```python
from build123d import *

# Parameters (mm, degrees)
SKETCH3_R          = 8.5
SKETCH2_R          = 7.5
SKETCH4_W          = 13.98
SKETCH4_H          = 8.5
CUT_EXTRUDE1_DEPTH = 10
CUT_EXTRUDE2_DEPTH = 10
SKETCH6_R          = 1.25
CUT_EXTRUDE3_DEPTH = 10
CUT_EXTRUDE4_DEPTH = 12
FILLET1_R          = 1


with BuildPart() as part:
    # Sketch3 → Loft1 section 0
    with BuildSketch(Plane(origin=(0, 0, 0), x_dir=(0, 0, -1), z_dir=(1, 0, 0))):
        Circle(SKETCH3_R)
    # Sketch2 → Loft1 section 1
    with BuildSketch(Plane(origin=(-22, 0, 0), x_dir=(0, 0, -1), z_dir=(1, 0, 0))):
        Circle(SKETCH2_R)
    loft()

    # Sketch4 → Cut-Extrude1 (cut, symmetric)
    with BuildSketch(Plane.XY):
        with Locations((-17.99, 0)):
            Rectangle(SKETCH4_W, SKETCH4_H)
    extrude(amount=CUT_EXTRUDE1_DEPTH, both=True, mode=Mode.SUBTRACT)

    # Sketch5 → Cut-Extrude2 (cut, symmetric)
    with BuildSketch(Plane(origin=(0, 0, 0), x_dir=(1, 0, 0), z_dir=(0, 1, 0))):
        with BuildLine():
            Line((-23, -6.043769414), (-23.024844237, -1.493837243))
            ThreePointArc((-23.024844237, -1.493837243), (-21.216174997, 3.738120473), (-16.53, 6.685056145))
            Line((-16.53, 6.685056145), (-11, 6.777720856))
            Line((-11, 6.777720856), (-11, 10.146746938))
            Line((-11, 10.146746938), (-27.92, 10.146746938))
            Line((-27.92, 10.146746938), (-27.92, -8.723253062))
            Line((-27.92, -8.723253062), (-11, -8.723253062))
            Line((-11, -8.723253062), (-11, -6.777720856))
            Line((-11, -6.777720856), (-23, -6.043769414))
        make_face()
    extrude(amount=CUT_EXTRUDE2_DEPTH, both=True, mode=Mode.SUBTRACT)

    # Sketch6 → Cut-Extrude3 (cut, symmetric)
    with BuildSketch(Plane(origin=(0, 0, 0), x_dir=(1, 0, 0), z_dir=(0, 1, 0))):
        with Locations((-15.3, 0.5)):
            Circle(SKETCH6_R)
    extrude(amount=CUT_EXTRUDE3_DEPTH, both=True, mode=Mode.SUBTRACT)

    # Sketch8 → Cut-Extrude4 (cut)
    with BuildSketch(Plane(origin=(0, 0, 0), x_dir=(0, 0, -1), z_dir=(1, 0, 0))):
        with BuildLine():
            Line((-4.5, 4.25), (4.5, 4.25))
            ThreePointArc((4.5, 4.25), (5.333449887, -0.025663938), (4.27, -4.25))
            Line((4.27, -4.25), (-4.73, -4.25))
            ThreePointArc((-4.73, -4.25), (-5.563449887, 0.025663938), (-4.5, 4.25))
        make_face()
    extrude(amount=-CUT_EXTRUDE4_DEPTH, mode=Mode.SUBTRACT)

    # Fillet1
    fillet1_edges = [part.edges().sort_by_distance(p)[0] for p in [
        (-22, -4.303290893, 6.104932034),
        (-22, 4.303290893, 6.104932034),
    ]]
    fillet(fillet1_edges, radius=FILLET1_R)


solid = part.part
```
CAD build for the part. Positions are in the model's coordinates, mm. A direction names the side the tool comes from. Coordinates: 2 decimals unless noted, no trailing zeros. Loops run counter-clockwise (first coordinate to the right, second up) from the corner with the lowest first, then second, coordinate; pieces in that order, holes last. Notation, with made-up numbers: (-34.75, 55) - (-7.75, 55) arc R15 cw to (-7.75, 80) - close; hole circle Ø5 at (-19.5, -15). An arc over 180 degrees is marked (long way). Return JSON: item names as keys, results as strings.
1. Band-saw the part on C-C (x = -15.25). Give the cut face in (y, z), and give its area (3 significant figures).
Result:
{"outline": "(-7.77, 0.75) - (-4.25, 0.75) - (-4.25, 6.52) - (-4.3, 6.52) arc R7.81 ccw to start; (-7.61, -1.75) arc R7.81 ccw to (-4.25, -6.55) - (-4.25, -1.75) - close; (4.25, -6.55) arc R7.81 ccw to (7.61, -1.75) - (4.25, -1.75) - close; (4.25, 0.75) - (7.77, 0.75) arc R7.81 ccw to (4.3, 6.52) - (4.25, 6.52) - close", "area": "48.1 mm2"}
2. Mould opens along Z. For faces 1 (the cylindrical face through (-14.723, 6.079, 0.609)), 2 (the flat face through (0, -6, 0)), 3 (the cylindrical face through (-21, 5, -4)), 4 (the conical face through (-11.154, -4.864, 6.343)) say: released by +Z, released by -Z, zero draft, split by the parting line, or undercut.
Result:
{"face 1": "undercut", "face 2": "zero draft", "face 3": "released by -Z", "face 4": "split by the parting line"}
3. Drop flat-ended pins along their axis: pin 1 (1 mm diameter, centred on x = -18, z = -6, fed in from +Y); pin 2 (10 mm diameter, centred on x = -9.5, z = -4, fed in from +Y); pin 3 (2 mm diameter, centred on x = -5.5, z = 1, fed in from -Y); pin 4 (3 mm diameter, centred on x = -17, y = -2, fed in from +Z). Give the stop position or say it passes through.
Result:
{"pin 1": "stops at y = 5.36", "pin 2": "stops at y = 8.22", "pin 3": "stops at y = -8.28", "pin 4": "passes through"}
4. 3-axis set-ups, long thin cutter, end or side, ignore diameter. For faces 5 (the flat face through (-22, -6, 1)), 6 (the cylindrical face through (-5.423, -0.036, 5.565)), 7 (the flat face through (-11, 4.25, 0)), 8 (the flat face through (-11, 0, 7)): which of +Z, -Z, +X, -X, +Y, -Y reach the whole face in a straight line?
Result:
{"face 5": "+Z, -Z, -X, +Y, -Y", "face 6": "+X, -X", "face 7": "-X", "face 8": "+Z, -Z, -X"}
5. Band-saw the part on D-D (x = -9.25). Give the cut face in (y, z).
Result:
{"outline": "circle Ø16.16 at (0, 0); hole (-4.25, -4.27) arc R10 ccw to (4.25, -4.5) - (4.25, 4.5) arc R10 ccw to (-4.25, 4.73) - close"}
6. Probe L1, parallel to X at y = 5.65, z = -0.5; L2, parallel to Y at x = -16.5, z = 4.25; L3, parallel to X at y = 0, z = -6.75. List the from-to ranges inside material, lowest first. Write a range as from..to.
Result:
{"L1": "x = -22..-16.55, -14.05..0", "L2": "y = -6.48..-4.25, 4.25..6.48", "L3": "x = -11..0"}
7. Band-saw the part on B-B (z = 0). Give the cut face in (x, y), and give its area (3 significant figures).
Result:
{"outline": "(-22, -7.5) - (-16.45, -7.75) - (-16.45, -4.25) - (-22, -4.25) - close; (-22, 4.25) - (-16.45, 4.25) - (-16.45, 7.75) - (-22, 7.5) - close; (-14.15, -7.86) - (0, -8.5) - (0, -4.25) - (-14.15, -4.25) - close; (-14.15, 4.25) - (0, 4.25) - (0, 8.5) - (-14.15, 7.86) - close", "area": "149 mm2"}
